Input: dimensioned drawing with shaded views. Units: mm. Origin: part minimum x, y, z. A direction names the side the tool comes from. Give positions to 0.01 mm unless a question says otherwise; leave off trailing zeros. Order: outer loops, then holes, each group sorted by start corner. A loop starts at its lowest first (then second) coordinate and runs counter-clockwise, first axis right, second up. Notation, with made-up numbers: (-2, -2.75) -> (34, -2.75) arc R25 ccw to (34, 26.25) -> close; hole circle Ø6 at (68, -17). An arc over 180 degrees is marked (long way). One line per question, with ' | ' between items. Start each with the question number.
(1) Section B-B (x = 6.55). Return loops of the section in (y, z), then the cut area to 3 significant figures.
(2) Set-up query: the marked faces 1, 2 and 3. Return all of +Z, -Z, +X, -X, +Y, -Y with unobstructed straight access to the full face (end or side cutting, diameter ignored); none if empty.
(3) Ray query, L1, parallel to Y at x = 6, z = 3.5; L2, parallel to X at y = 2, z = 9.75; L3, parallel to Y at x = 16.25, z = 9. Return the intervals inside material, ascending.
(4) First-contact query: pin 1 Ø1 at (x, y) = (8, 14) entering from -Z; pin 2 Ø1.2 at (x, z) = (14, 6.5) entering from -Y; pin 3 Ø2 at (x, z) = (14.5, 7.5) entering from +Y. Flat tips, straight axial feed; report the tip coordinate or a pass-through.
(5) Section A-A (z = 9.3). Return loops of the section in (x, y).
(6) Section D-D (x = 15.75). Return loops of the section in (y, z), then the cut area to 3 significant figures.
(7) Section C-C (y = 16.25). Return loops of the section in (x, z), then the cut area to 3 significant figures.
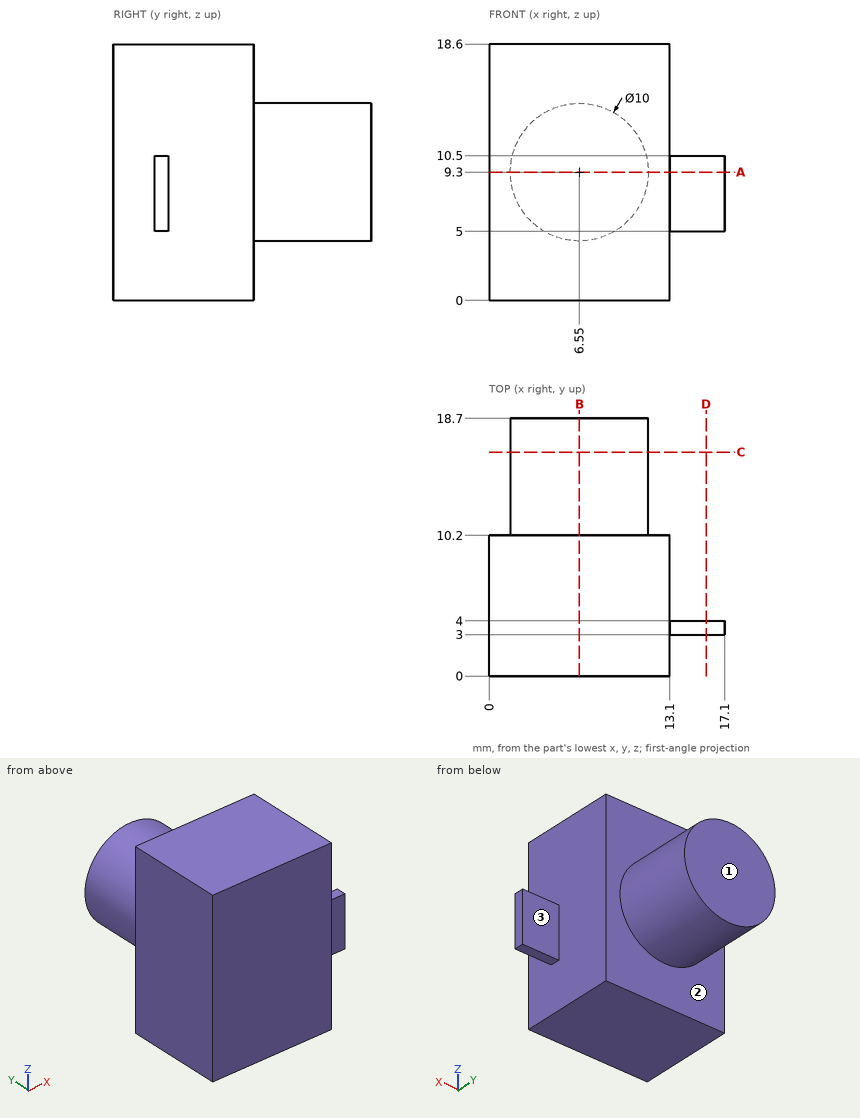
Response:
1) outline: (0, 0) -> (10.2, 0) -> (10.2, 4.3) -> (18.7, 4.3) -> (18.7, 14.3) -> (10.2, 14.3) -> (10.2, 18.6) -> (0, 18.6) -> close | area: 275 mm^2
2) face 1: +Z, -Z, +X, -X, +Y | face 2: +Y | face 3: +Z, -Z, +X, +Y
3) L1: y = 0 to 10.2 | L2: x = 0 to 13.1 | L3: y = 3 to 4
4) pin 1: stops at z = 4.39 | pin 2: stops at y = 3 | pin 3: stops at y = 4
5) outline: (0, 0) -> (13.1, 0) -> (13.1, 3) -> (17.1, 3) -> (17.1, 4) -> (13.1, 4) -> (13.1, 10.2) -> (11.55, 10.2) -> (11.55, 18.7) -> (1.55, 18.7) -> (1.55, 10.2) -> (0, 10.2) -> close
6) outline: (3, 5) -> (4, 5) -> (4, 10.5) -> (3, 10.5) -> close | area: 5.50 mm^2
7) outline: circle Ø10 at (6.55, 9.3) | area: 78.5 mm^2
